```python
from build123d import *

# Parameters (mm, degrees)
F0_W     = 2.581628
F0_H     = 0.791415
F0_W_2   = 2.597917
F0_H_2   = 1.066693
F0_W_3   = 2.718348
F0_H_3   = 1.806498
F0_R     = 5.178657
F0_W_4   = 9.823907
F0_H_4   = 2.942012
F1_DEPTH = 1.2


with BuildPart() as f1:
    # F0 (on Top) → F1 (new body)
    with BuildSketch(Plane.XY):
        with BuildLine():
            Line((-6.29297, -85.910204), (-6.29297, 54.089796))
            ThreePointArc((-6.29297, 54.089796), (-26.288129, 74.529796), (-46.283289, 54.089796))
            Line((-46.283289, 54.089796), (-46.283289, -85.910204))
            Line((-46.283289, -85.910204), (-6.29297, -85.910204))
        make_face()
        with Locations((-37.201445, -61.692785)):
            Rectangle(F0_W, F0_H, mode=Mode.SUBTRACT)
        with Locations((-37.210507, -59.800263)):
            Rectangle(F0_W_2, F0_H_2, mode=Mode.SUBTRACT)
        with Locations((-37.081471, -57.331383)):
            Rectangle(F0_W_3, F0_H_3, mode=Mode.SUBTRACT)
        with BuildLine():
            Line((-35.481431, -55.46467), (-38.199779, -55.46467))
            Line((-38.199779, -55.46467), (-38.199779, -53.967856))
            Line((-38.199779, -53.967856), (-35.309382, -53.967856))
            add(Edge.make_bspline(
                [(-35.309382, -53.967856), (-35.429817, -54.260336), (-35.481431, -54.982934), (-35.481431, -55.46467)],
                knots=[0, 0, 0, 0, 1.50667, 1.50667, 1.50667, 1.50667], degree=3))
        make_face(mode=Mode.SUBTRACT)
        with BuildLine():
            Line((-35.155974, -53.070802), (-37.735078, -53.070802))
            add(Edge.make_bspline(
                [(-36.615845, -48.277561), (-37.310701, -49.868666), (-37.715785, -51.382598), (-37.735078, -53.070802)],
                knots=[0, 0, 0, 0, 4.922179, 4.922179, 4.922179, 4.922179], degree=3))
            Line((-36.615845, -48.277561), (-33.963747, -48.277561))
            add(Edge.make_bspline(
                [(-33.963747, -48.277561), (-34.742344, -49.834754), (-34.912664, -51.440611), (-35.155974, -53.070802)],
                knots=[0, 0, 0, 0, 4.939288, 4.939288, 4.939288, 4.939288], degree=3))
        make_face(mode=Mode.SUBTRACT)
        with BuildLine():
            add(Edge.make_bspline(
                [(-33.896647, -42.036764), (-34.845561, -43.812942), (-35.697155, -45.613449), (-36.281101, -47.389627)],
                knots=[0, 0, 0, 0, 5.859928, 5.859928, 5.859928, 5.859928], degree=3))
            Line((-33.896647, -42.036764), (-30.660599, -42.036764))
            add(Edge.make_bspline(
                [(-30.660599, -42.036764), (-31.779833, -43.983262), (-32.801744, -45.516126), (-33.38569, -47.389627)],
                knots=[0, 0, 0, 0, 6.006601, 6.006601, 6.006601, 6.006601], degree=3))
            Line((-33.38569, -47.389627), (-36.281101, -47.389627))
        make_face(mode=Mode.SUBTRACT)
        with BuildLine():
            Line((-29.023839, -53.121161), (-27.305199, -55.41268))
            ThreePointArc((-27.305199, -55.41268), (-25.748689, -59.722554), (-24.440799, -55.330839))
            Line((-24.440799, -55.330839), (-22.865377, -53.121161))
            ThreePointArc((-22.865377, -53.121161), (-25.944608, -62.574254), (-29.023839, -53.121161))
        make_face(mode=Mode.SUBTRACT)
        with Locations((-25.738571, -46.987876)):
            Circle(F0_R, mode=Mode.SUBTRACT)
        with BuildLine():
            add(Edge.make_bspline(
                [(-17.875146, -19.652883), (-18.462803, -23.768686), (-20.271629, -27.596692), (-22.875761, -31.155674)],
                knots=[0, 0, 0, 0, 12.542741, 12.542741, 12.542741, 12.542741], degree=3))
            Line((-17.875146, -19.652883), (-15.126339, -19.652883))
            add(Edge.make_bspline(
                [(-15.126339, -19.652883), (-15.713997, -24.289511), (-18.029595, -29.035197), (-21.1288, -33.232335)],
                knots=[0, 0, 0, 0, 14.846921, 14.846921, 14.846921, 14.846921], degree=3))
            ThreePointArc((-21.1288, -33.232335), (-20.771988, -34.290864), (-20.651166, -35.401359))
            ThreePointArc((-20.651166, -35.401359), (-23.323252, -39.924203), (-28.57408, -39.766207))
            add(Edge.make_bspline(
                [(-28.57408, -39.766207), (-29.019574, -40.191628), (-29.530527, -40.629588), (-29.760677, -41.22673)],
                knots=[0, 0, 0, 0, 1.881791, 1.881791, 1.881791, 1.881791], degree=3))
            Line((-29.760677, -41.22673), (-33.001378, -41.22673))
            add(Edge.make_bspline(
                [(-30.314623, -37.934667), (-31.40403, -39.169718), (-32.42594, -40.264621), (-33.001378, -41.22673)],
                knots=[0, 0, 0, 0, 4.249274, 4.249274, 4.249274, 4.249274], degree=3))
            ThreePointArc((-30.314623, -37.934667), (-29.293093, -31.584655), (-22.875761, -31.155674))
        make_face(mode=Mode.SUBTRACT)
        with BuildLine():
            Line((-30.725121, -25.672881), (-24.253521, -25.672881))
            ThreePointArc((-24.253521, -25.672881), (-23.118539, -23.782431), (-24.45812, -22.031))
            Line((-24.45812, -22.031), (-30.725121, -22.031))
            Line((-30.725121, -22.031), (-30.725121, -19.453041))
            Line((-30.725121, -19.453041), (-24.45812, -19.453041))
            ThreePointArc((-24.45812, -19.453041), (-20.744201, -23.754778), (-24.253521, -28.224992))
            Line((-24.253521, -28.224992), (-30.725121, -28.224992))
            Line((-30.725121, -28.224992), (-30.725121, -25.672881))
        make_face(mode=Mode.SUBTRACT)
        with Locations((-25.720231, -15.450788)):
            Rectangle(F0_W_4, F0_H_4, mode=Mode.SUBTRACT)
        Polygon((-30.681022, -11.994411), (-30.681022, -3.235085), (-28.346451, -3.235186), (-28.346451, -6.20359), (-20.755121, -6.20359), (-20.755121, -8.953013), (-28.346451, -8.953013), (-28.346451, -11.994411), align=None, mode=Mode.SUBTRACT)
        Polygon((-30.762237, -1.389609), (-30.762237, 1.597551), (-23.723995, 1.597551), (-23.723995, 6.303352), (-20.982355, 6.303352), (-20.982355, -1.389609), align=None, mode=Mode.SUBTRACT)
        Polygon((-30.632185, 14.041182), (-20.982355, 18.198028), (-20.982355, 15.322189), (-22.808162, 14.535688), (-22.808162, 10.689207), (-20.982355, 10.095867), (-20.982355, 7.108707), (-30.632185, 11.118867), align=None, mode=Mode.SUBTRACT)
        Polygon((-20.763781, 22.507036), (-20.763781, 19.669064), (-30.717358, 19.669064), (-30.717358, 22.507036), (-27.090734, 24.833532), (-30.717358, 27.049802), (-30.717358, 30.087957), (-20.763781, 30.087957), (-20.763781, 27.049802), (-26.145658, 27.049802), (-22.519033, 24.833532), (-26.145658, 22.507036), align=None, mode=Mode.SUBTRACT)
    extrude(amount=F1_DEPTH)


solid = f1.part
```
Build history of the part. All positions in model axes, mm. A direction names the side the tool comes from. Coordinates: 2 decimals unless noted, no trailing zeros. Write each loop counter-clockwise with the first axis right and the second up, starting at its lowest first coordinate (ties: lowest second). Pieces come first, ordered by that corner, then holes.
1. Drop flat-ended pins along their axis: pin 1 (4 mm diameter, centred on x = -35, y = -34.5, fed in from -Z); pin 2 (0.6 mm diameter, centred on y = 28, z = 0.5, fed in from +X); pin 3 (8.5 mm diameter, centred on x = -25.74, y = -46.99, fed in from +Z). Give the stop position or say it passes through.
Answer block:
pin 1: stops at z = 0
pin 2: stops at x = -6.29
pin 3: passes through
2. Pull direction Y, two halves, no side cores. Call faces 1 (the cylindrical face through (-25.833, -59.723, 0.592)), 2 (the flat face through (-27, -5, 1.2)): released by +Y, released by -Y, zero draft, split by the parting line, or undercut.
Answer block:
face 1: undercut
face 2: zero draft
3. Drill centre lines: probe 1 along X at (y, z) = (28, 0.1); probe 2 along X at (y, z) = (-56, 0.6); probe 3 along X at (y, z) = (-48.5, 1.05). Where is each one in solid material? Low to high.
Answer block:
probe 1: x = -46.28 to -30.72, -20.76 to -6.29
probe 2: x = -46.28 to -31, -27.84 to -23.79, -20.89 to -6.29
probe 3: x = -46.28 to -36.71, -34.07 to -30.69, -20.79 to -6.29
4. Band-saw the part on C-C, the plane x = -10.5. Give the cut face in (y, z), and give its area (3 significant figures).
Answer block:
outline: (-85.91, 0) - (66.81, 0) - (66.81, 1.2) - (-85.91, 1.2) - close
area: 183 mm2
5. 3-axis set-ups, long thin cutter, end or side, ignore diameter. For faces 3 (the cylindrical face through (-20.747, -23.669, 0.592)), 4 (the flat face through (-27, -5, 0)): which of +Z, -Z, +X, -X, +Y, -Y reach the whole face in a straight line?
Answer block:
face 3: +Z, -Z
face 4: -Z, +X, -X, +Y, -Y
6. Band-saw the part on A-A, the plane y = 12.5. Give the cut face in (x, z), and give its area (3 significant figures).
Answer block:
outline: (-46.28, 0) - (-30.63, 0) - (-30.63, 1.2) - (-46.28, 1.2) - close; (-22.81, 0) - (-6.29, 0) - (-6.29, 1.2) - (-22.81, 1.2) - close
area: 38.6 mm2
7. Band-saw the part on B-B, the plane z = 0.7. Give the number of separate pieces and of enclosed holes in the cut face, and give its area (3 significant figures).
Answer block:
separate pieces: 1
enclosed holes: 15
area: 5,630 mm2
